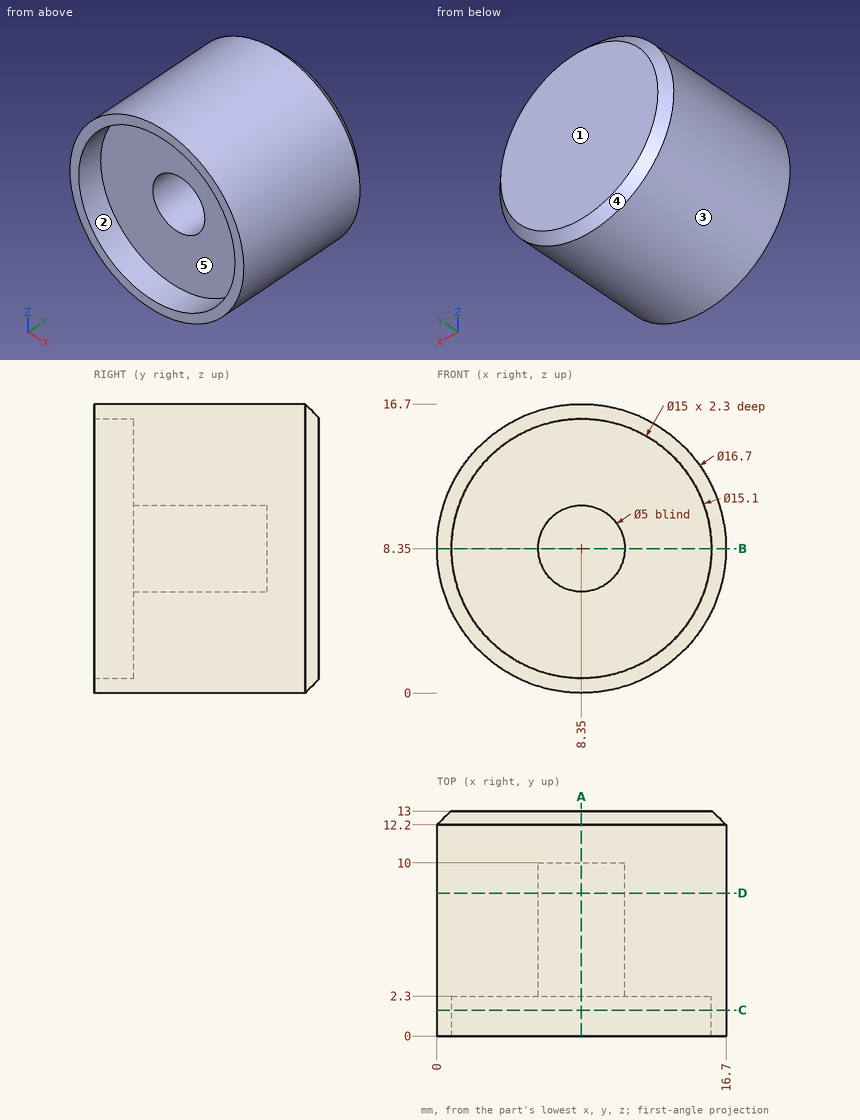
For this review, use the dimensioned drawing (mm, ordinates from the lowest corner) and the shaded views. A direction names the side the tool comes from. Coordinates: 2 decimals unless noted, no trailing zeros. Write each loop counter-clockwise with the first axis right and the second up, starting at its lowest first coordinate (ties: lowest second). Pieces come first, ordered by that corner, then holes. Notation, with made-up numbers: (71.25, -28) - (81.25, -28) arc R9 cw to (81.25, -23) - close; hole circle Ø3 at (17, 41.5). An arc over 180 degrees is marked (long way). Answer in a Markdown table with one row per item. Add a question column.
Q1. To check wall thickness, follow line 1 along X through (y, z) = (1.25, 8.35); line 2 along X through (y, z) = (5, 8.35); line 3 along Z through (x, y) = (14.25, 1). State the ranges of each line that lie inside material, in increasing order. Write a range as from..to.
Q2. Consider section B-B on z = 8.35. Give the boundary of the cut face in (x, y), then the cut area to 3 significant figures.
Q3. Consider section D-D on y = 8.25. Give the boundary of the cut face in (x, z).
Q4. For the marked faces 4 and 5, list the 3-axis set-ups (+Z, -Z, +X, -X, +Y, -Y) from which the entire face can be reached by the end or side of a thin tool; tool diameter is ignored.
Q5. Consider section C-C on y = 1.5. Give the boundary of the cut face in (x, z).
Q6. Consider section A-A on x = 8.35. Give the boundary of the cut face in (y, z), then the cut area to 3 significant figures.
Q7. Draft analysis for pull direction Z (two halves, no side actions). For the marked faces 1, 2 and 3, state which applies: +Z half, -Z half, draft (parallel to the pull), parting line (faces both ways), or undercut.
Q8. Clearance check with flat-ended pins moving along their axes: pin 1 (6 mm diameter, centred on y = 4, z = 3, fed in from +X); pin 2 (4 mm diameter, centred on x = 8, z = 9.5, fed in from -Y); pin 3 (1.5 mm diameter, centred on x = 2, y = 3.5, fed in from -Z). State where each tip first meets the part, or that it passes through.
Answers below:
| question | item | result |
|---|---|---|
| 1 | line 1 | 0..0.85, 15.85..16.7 |
| 1 | line 2 | 0..5.85, 10.85..16.7 |
| 1 | line 3 | 2.44..3.72, 12.98..14.26 |
| 2 | outline | (0, 0) - (0.85, 0) - (0.85, 2.3) - (5.85, 2.3) - (5.85, 10) - (10.85, 10) - (10.85, 2.3) - (15.85, 2.3) - (15.85, 0) - (16.7, 0) - (16.7, 12.2) - (15.9, 13) - (0.8, 13) - (0, 12.2) - close |
| 2 | area | 143 mm² |
| 3 | outline | circle Ø16.7 at (8.35, 8.35); hole circle Ø5 at (8.35, 8.35) |
| 4 | face 4 | +Y |
| 4 | face 5 | -Y |
| 5 | outline | circle Ø16.7 at (8.35, 8.35); hole circle Ø15 at (8.35, 8.35) |
| 6 | outline | (0, 0) - (12.2, 0) - (13, 0.8) - (13, 15.9) - (12.2, 16.7) - (0, 16.7) - (0, 15.85) - (2.3, 15.85) - (2.3, 10.85) - (10, 10.85) - (10, 5.85) - (2.3, 5.85) - (2.3, 0.85) - (0, 0.85) - close |
| 6 | area | 143 mm² |
| 7 | face 1 | draft |
| 7 | face 2 | undercut |
| 7 | face 3 | parting line |
| 8 | pin 1 | x = 16.36 |
| 8 | pin 2 | y = 2.3 |
| 8 | pin 3 | z = 2.16 |
